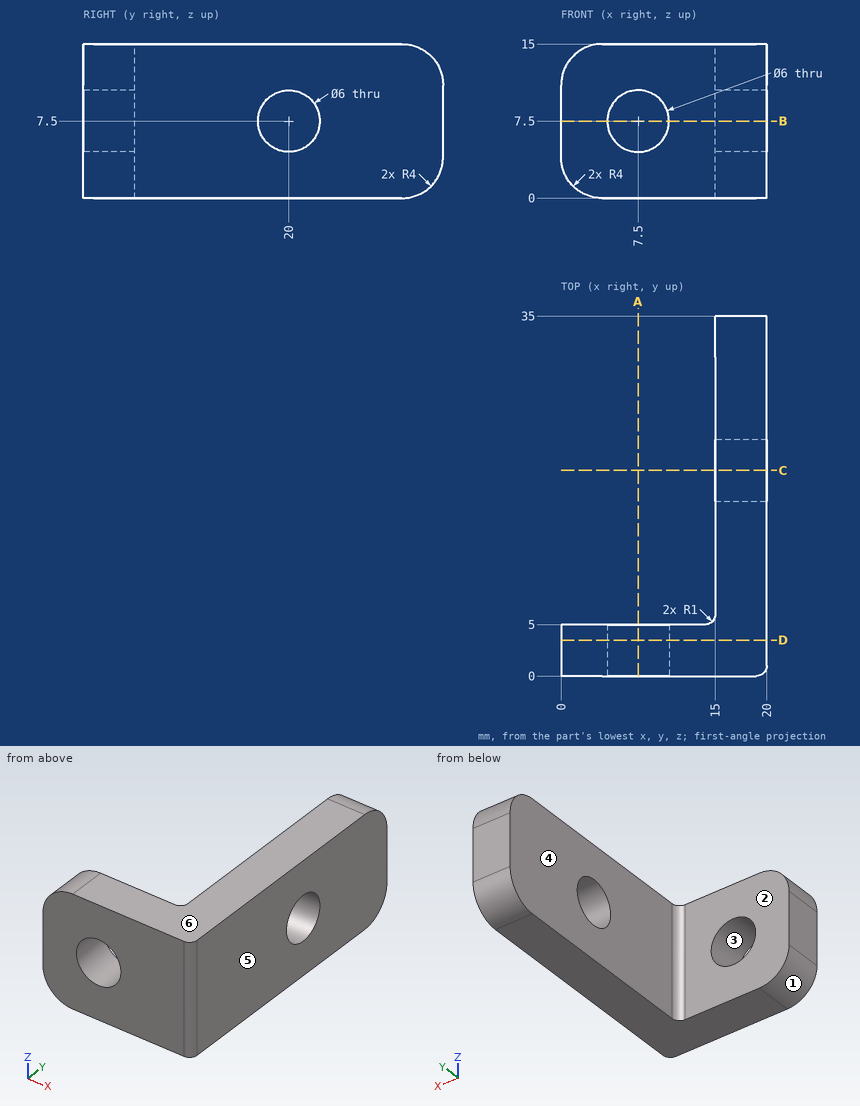
Here's the drawing with two shaded views (mm, measured from the low corner). I have some questions. A direction names the side the tool comes from. Round coordinates to 2 decimals unless told otherwise and drop trailing zeros. Loops run counter-clockwise (first coordinate to the right, second up) from the corner with the lowest first, then second, coordinate; pieces in that order, holes last. Notation, with made-up numbers: M -8,-33.5 L 17,-33.5 A30 cw 17,2.5 Z; hole C -17,-23.5 d6. An arc over 180 degrees is marked long. Answer as a JSON object with one key per item and string values. Group by question number.
Q1. We'd pull the mould along X, two halves only. Please class the marked faces 3, 4, 5 and 6: +X half, -X half, draft (parallel to the pull), parting line (faces both ways), or undercut.
Q2. On a 3-axis mill with a long thin cutter (end or side, diameter ignored), from which of +Z, -Z, +X, -X, +Y, -Y can I reach the whole of each face in a straight line? I mean the marked faces 1 and 2. Say none if no direction works.
Q3. Imagine slicing it at C-C, the plane y = 20. Please give me the cut outline in (x, z), then the cut area to 3 significant figures.
Q4. Imagine slicing it at D-D, the plane y = 3.5. Please give me the cut outline in (x, z), then the cut area to 3 significant figures.
Q5. Will these pins go through, and if not, where does the flat tip stop? pin 1 (7.5 mm diameter, centred on y = 20, z = 11, fed in from -X); pin 2 (4 mm diameter, centred on x = 4, z = 9.5, fed in from +Y); pin 3 (10 mm diameter, centred on x = 4.5, y = 9.5, fed in from +Z).
Q6. Imagine slicing it at B-B, the plane z = 7.5. Please give me the cut outline in (x, y), then the cut area to 3 significant figures.
Q7. Please list where these lines run through material, in increasing order: L1, parallel to Z at x = 7.5, y = 1.65; L2, parallel to Y at x = 13.75, z = 5.75; L3, parallel to X at y = 27, z = 13.5.
Q8. Imagine slicing it at A-A, the plane x = 7.5. Please give me the cut outline in (y, z), then the cut area to 3 significant figures.
Findings:
{
 "1": {"face 3": "undercut", "face 4": "-X half", "face 5": "+X half", "face 6": "draft"},
 "2": {"face 1": "-Z, -X, +Y, -Y", "face 2": "+Z, -Z, -X, +Y"},
 "3": {"outline": "M 15,0 L 20,0 L 20,4.5 L 15,4.5 Z; M 15,10.5 L 20,10.5 L 20,15 L 15,15 Z", "area": "45.0 mm2"},
 "4": {"outline": "M 0,4 A4 ccw 4,0 L 20,0 L 20,15 L 4,15 A4 ccw 0,11 Z; hole C 7.5,7.5 d6", "area": "265 mm2"},
 "5": {"pin 1": "stops at x = 15", "pin 2": "stops at y = 5", "pin 3": "stops at z = 15"},
 "6": {"outline": "M 0,0 L 4.5,0 L 4.5,5 L 0,5 Z; M 10.5,0 L 19,0 A1 ccw 20,1 L 20,17 L 15,17 L 15,6 A1 cw 14,5 L 10.5,5 Z; M 15,23 L 20,23 L 20,35 L 15,35 Z", "area": "190 mm2"},
 "7": {"L1": "z = 0 to 4.5, 10.5 to 15", "L2": "y = 0 to 5", "L3": "x = 15 to 20"},
 "8": {"outline": "M 0,0 L 5,0 L 5,4.5 L 0,4.5 Z; M 0,10.5 L 5,10.5 L 5,15 L 0,15 Z", "area": "45.0 mm2"}
}
